Geometry check sheet. Reference: drawing and pictorial views, mm from the part's lowest x, y, z. Round coordinates to 2 decimals unless told otherwise and drop trailing zeros. Loops run counter-clockwise (first coordinate to the right, second up) from the corner with the lowest first, then second, coordinate; pieces in that order, holes last. Notation, with made-up numbers: (23, 71.5) - (81, 71.5) arc R11 cw to (81, 91.5) - close; hole circle Ø3 at (-39, 19.5). An arc over 180 degrees is marked (long way). Answer in a Markdown table with one row per item. Add a question column.
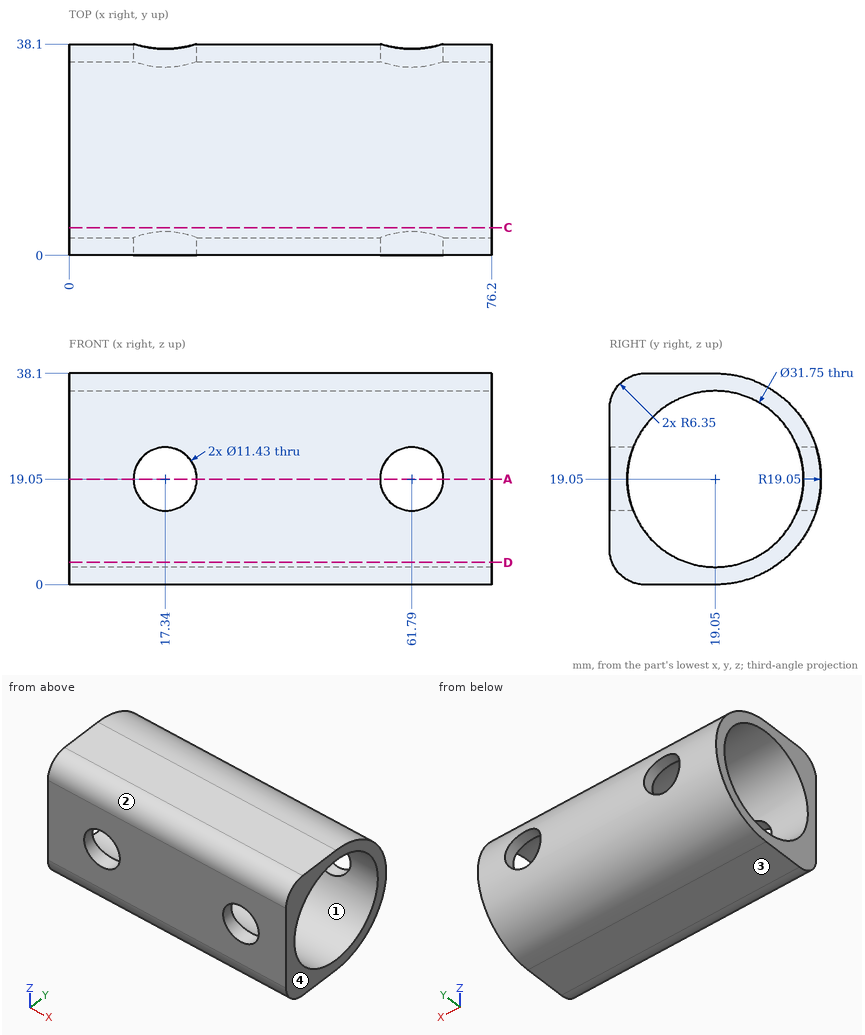
Q1. Cross-section at A-A, the plane z = 19.05. Enter the section's corners in (x, y) (1 decimal).
Q2. Scan lines: line 1 (X direction, y = 2, z = 19) (1 decimal); line 2 (Z direction, x = 28, y = 29) (1 decimal); line 3 (Z direction, x = 14, y = 36.5). Record each from-to range of solid material in increasing order. Write a range as from..to.
Q3. Cross-section at D-D, the plane z = 4. Enter the section's corners in (x, y), plus the area to 3 significant figures.
Q4. Cross-section at C-C, the plane y = 5. Enter the section's corners in (x, z) (1 decimal).
Q5. Depth check by flat-ended pin: P1, Ø12, axis at x = 30.5, y = 30.5, coming from the -Z side; P2, Ø18.5, axis at x = 61.79, z = 19.05, coming from the +Y side; P3, Ø3, axis at x = 26, z = 10.5, coming from the +Y side; P4, Ø1, axis at x = 23, z = 25.5, coming from the +Y side. Enter the tip coordinate at first touch or a pass-through.
Q6. Release check for a two-part mould opening along Z. For the marked faces 1, 2, 3 and 4 record: +Z half, -Z half, draft (parallel to the pull), parting line (faces both ways), or undercut.
Check sheet entries:
| question | item | result |
|---|---|---|
| 1 | outline | (0, 0) - (11.6, 0) - (11.6, 3.2) - (0, 3.2) - close; (0, 34.9) - (11.6, 34.9) - (11.6, 38.1) - (0, 38.1) - close; (23.1, 0) - (56.1, 0) - (56.1, 3.2) - (23.1, 3.2) - close; (23.1, 34.9) - (56.1, 34.9) - (56.1, 38.1) - (23.1, 38.1) - close; (67.5, 0) - (76.2, 0) - (76.2, 3.2) - (67.5, 3.2) - close; (67.5, 34.9) - (76.2, 34.9) - (76.2, 38.1) - (67.5, 38.1) - close |
| 2 | line 1 | 0..11.6, 23.1..56.1, 67.5..76.2 |
| 2 | line 2 | 2.8..6.7, 31.4..35.3 |
| 2 | line 3 | 11.41..14.41, 23.69..26.69 |
| 3 | outline | (0, 0.45) - (76.2, 0.45) - (76.2, 14) - (0, 14) - close; (0, 24.1) - (76.2, 24.1) - (76.2, 30.73) - (0, 30.73) - close |
| 3 | area | 1,540 mm² |
| 4 | outline | (0, 0.1) - (76.2, 0.1) - (76.2, 11.7) - (0, 11.7) - close; (0, 26.4) - (76.2, 26.4) - (76.2, 38) - (0, 38) - close |
| 5 | P1 | z = 0.8 |
| 5 | P2 | y = 38.1 |
| 5 | P3 | y = 36.75 |
| 5 | P4 | y = 37.15 |
| 6 | face 1 | undercut |
| 6 | face 2 | +Z half |
| 6 | face 3 | -Z half |
| 6 | face 4 | draft |
